Verification items for the finished model (mm, model axes). Face numbers are marked on the shaded views. A direction names the side the tool comes from. Give positions to 0.01 mm unless a question says otherwise; leave off trailing zeros. Order: outer loops, then holes, each group sorted by start corner. A loop starts at its lowest first (then second) coordinate and runs counter-clockwise, first axis right, second up.
(1) Access from +Z, -Z, +X, -X, +Y, -Y to the whole of each face (thin tool, end or side, straight path). Record for the marked faces 1 and 2.
(2) Scan lines: L1, parallel to X at y = 1, z = 18; L2, parallel to Y at x = 97.95, z = 61.1; L3, parallel to X at y = 3, z = 17 (3 decimals). Record each from-to range of solid material in increasing order.
(3) Sectioned sample at C-C on z = 37.5. Record the cut outline in (x, y).
(4) Sectioned sample at D-D on x = 92. Record the cut outline in (y, z), plus the area to 3 significant figures.
(5) Gauge pin test, flat ends, axial feed: pin 1 (4.5 mm diameter, centred on x = 71.9, z = 58.1, fed in from -Y); pin 2 (6 mm diameter, centred on y = 14, z = 23.5, fed in from -X); pin 3 (2 mm diameter, centred on x = 87, z = 31, fed in from +Y). Record the tip position at first contact, or that the pin passes through.
(6) Sectioned sample at A-A on x = 18.9. Record the cut outline in (y, z).
(7) Sectioned sample at B-B on y = 12. Record the cut outline in (x, z), plus the area to 3 significant figures.
Autodesk Inventor part; units mm, degrees
ref_plane "YZ Plane" through (0, 0, 0) normal (1, 0, 0) x (0, 1, 0)
ref_plane "XZ Plane" through (0, 0, 0) normal (0, 1, 0) x (-1, 0, 0)
ref_plane "XY Plane" through (0, 0, 0) normal (0, 0, 1) x (1, 0, 0)
sketch "Sketch1" plane through (0, 0, 0) normal (0, 0, 1) x (1, 0, 0)
  line L0 (0, 0) -> (101.6, 0)
  line L1 (101.6, 0) -> (101.6, 50.8)
  line L2 (0, 0) -> (0, 4.7625)
  line L3 (0, 4.7625) -> (96.8375, 4.7625)
  line L4 (96.8375, 4.7625) -> (96.8375, 50.8)
  line L5 (96.8375, 50.8) -> (101.6, 50.8)
  dimension "d0" = 101.6
  dimension "d1" = 50.8
  dimension "d2" = 4.7625
extrude "Extrusion1" add sketch "Sketch1" along normal blind 76.2
sketch "Sketch2" plane through (0, 0, 0) normal (0, -1, 0) x (1, 0, 0)
  line L0 (18.9, 18.1) -> (71.9, 18.1) construction
  line L1 (71.9, 18.1) -> (71.9, 58.1) construction
  line L2 (71.9, 58.1) -> (18.9, 58.1) construction
  line L3 (18.9, 58.1) -> (18.9, 18.1) construction
  line L4 (101.6, 0) -> (101.6, 76.2) construction
  circle A0 centre (18.9, 58.1) radius 2.5
  circle A1 centre (18.9, 18.1) radius 2.5
  circle A2 centre (71.9, 58.1) radius 2.5
  circle A3 centre (71.9, 18.1) radius 2.5
  point P0 (0, 0)
  point P1 (45.4, 58.1)
  point P2 (71.9, 38.1)
  point P3 (101.6, 38.1)
  dimension "d5" = 53
  dimension "d6" = 40
  dimension "d7" = 56.2
  dimension "d8" = 5
extrude "Extrusion2" cut sketch "Sketch2" against normal up to surface (4.7625 mm away)
sketch "Sketch3" plane through (101.6, 0, 0) normal (1, 0, 0) x (0, 0, -1)
  line L0 (-15.1, 14.7625) -> (-61.1, 14.7625) construction
  line L1 (-61.1, 14.7625) -> (-61.1, 39.7625) construction
  line L2 (-61.1, 39.7625) -> (-15.1, 39.7625) construction
  line L3 (-15.1, 39.7625) -> (-15.1, 14.7625) construction
  line L4 (0, 0) -> (-76.2, 0) construction
  circle A0 centre (-15.1, 14.7625) radius 4
  circle A1 centre (-15.1, 39.7625) radius 4
  circle A2 centre (-61.1, 14.7625) radius 4
  circle A3 centre (-61.1, 39.7625) radius 4
  point P0 (0, 4.7625)
  point P1 (-38.1, 14.7625)
  point P2 (-38.1, 0)
  dimension "d11" = 46
  dimension "d12" = 25
  dimension "d13" = 10
  dimension "d14" = 8
extrude "Extrusion3" cut sketch "Sketch3" against normal blind 25.4
properties part number "L_Bracketr"
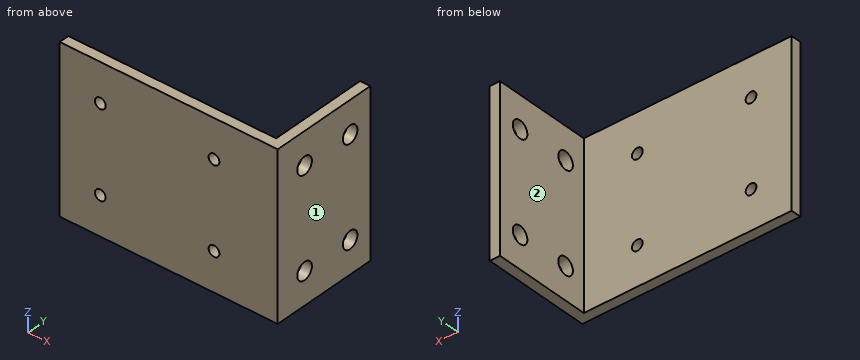
Ans:
1. face 1: +Z, -Z, +X, +Y, -Y
1. face 2: +Z, -Z, -X, +Y
2. L1: x = 0 to 16.4, 21.4 to 69.4, 74.4 to 101.6
2. L2: y = 0 to 10.76, 18.76 to 35.76, 43.76 to 50.8
2. L3: x = 0 to 16.655, 21.145 to 69.655, 74.145 to 101.6
3. outline: (0, 0) - (101.6, 0) - (101.6, 50.8) - (96.84, 50.8) - (96.84, 4.76) - (0, 4.76) - close
4. outline: (0, 0) - (4.76, 0) - (4.76, 76.2) - (0, 76.2) - close
4. area: 363 mm2
5. pin 1: passes through
5. pin 2: stops at x = 96.84
5. pin 3: stops at y = 4.76
6. outline: (0, 0) - (4.76, 0) - (4.76, 15.6) - (0, 15.6) - close; (0, 20.6) - (4.76, 20.6) - (4.76, 55.6) - (0, 55.6) - close; (0, 60.6) - (4.76, 60.6) - (4.76, 76.2) - (0, 76.2) - close
7. outline: (96.84, 0) - (101.6, 0) - (101.6, 12.21) - (96.84, 12.21) - close; (96.84, 17.99) - (101.6, 17.99) - (101.6, 58.21) - (96.84, 58.21) - close; (96.84, 63.99) - (101.6, 63.99) - (101.6, 76.2) - (96.84, 76.2) - close
7. area: 308 mm2
